Check sheet for the modelled part. Datum: model origin and axes. Units: mm. Face numbers are marked on the shaded views. Give positions to 0.01 mm unless a question says otherwise; leave off trailing zeros. Order: outer loops, then holes, each group sorted by start corner. A loop starts at its lowest first (then second) coordinate and runs counter-clockwise, first axis right, second up.
```python
from build123d import *

# Parameters (mm, degrees)
CHAMFER1_SIZE = 1
FILLET1_R     = 1


with BuildPart() as part:
    # Sketch1 → Revolve1 (revolve)
    with BuildSketch(Plane.XY, mode=Mode.PRIVATE) as revolve1_sk:
        Polygon((0, 5), (10, 5), (10, 7.5), (3, 7.5), (3, 10.5), (0, 10.5), align=None)
    revolve(revolve1_sk.sketch.rotate(Axis((0, 0, 0), (1, 0, 0)), 90), axis=Axis((0, 0, 0), (1, 0, 0)))

    # Chamfer1
    chamfer1_edges = [part.edges().sort_by_distance(p)[0] for p in [
        (0, 0, -10.5),
        (3, 0, -10.5),
        (10, 0, -7.5),
        (10, 0, -5),
        (0, 0, -5),
    ]]
    chamfer(chamfer1_edges, length=CHAMFER1_SIZE)

    # Fillet1
    fillet1_edges = [part.edges().sort_by_distance(p)[0] for p in [
        (3, 0, -7.5),
    ]]
    fillet(fillet1_edges, radius=FILLET1_R)


solid = part.part
```
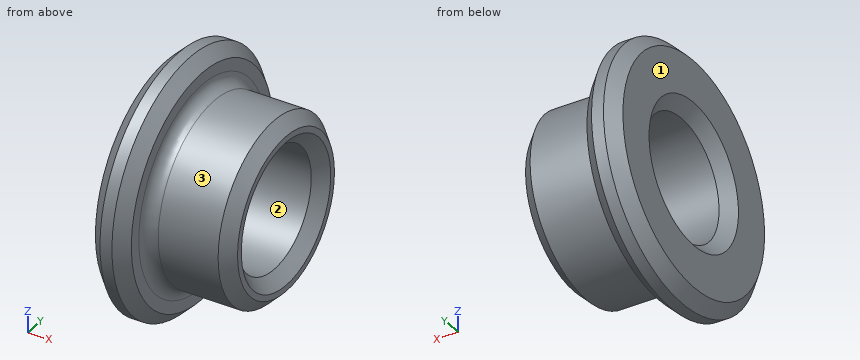
Q1. Material ranges on line 1 (Y direction, x = 1.5, z = 0); line 2 (Y direction, x = 4.5, z = 0); line 3 (X direction, y = -4.5, z = -7.25), recorded low to high.
Q2. Sectioned sample at C-C, the plane x = 2.5. Record the cut outline in (y, z), plus the area to 3 significant figures.
Q3. Sectioned sample at D-D, the plane x = 7. Record the cut outline in (y, z), plus the area to 3 significant figures.
Q4. Go/stop test with flat-tipped pins: P1, Ø6, axis at y = 0, z = 0, coming from the +X side; P2, Ø2, axis at x = 6.5, z = -2.5, coming from the +Y side; P3, Ø2, axis at x = 6.5, y = -2.5, coming from the +Z side; P4, Ø2, axis at x = 4.5, y = 1, coming from the -Z side. Record where each tip stops, or that it passes through.
Q5. Sectioned sample at A-A, the plane y = 0. Record the cut outline in (x, z), plus the area to 3 significant figures.
Q6. Draft check along Y on the marked faces 1, 2 and 3. Enter one of: pulls with the +Y half, pulls with the -Y half, needs draft (parallel to the pull), parting line crosses it, or undercut.
Filled in:
1. line 1: y = -10.5 to -5, 5 to 10.5
1. line 2: y = -7.5 to -5, 5 to 7.5
1. line 3: x = 0 to 3
2. outline: circle Ø20 at (0, 0); hole circle Ø10 at (0, 0)
2. area: 236 mm2
3. outline: circle Ø15 at (0, 0); hole circle Ø10 at (0, 0)
3. area: 98.2 mm2
4. P1: passes through
4. P2: stops at y = 7.35
4. P3: stops at z = 7.35
4. P4: stops at z = -7.58
5. outline: (0, -9.5) - (1, -10.5) - (2, -10.5) - (3, -9.5) - (3, -8.5) arc R1 cw to (4, -7.5) - (9, -7.5) - (10, -6.5) - (10, -6) - (9, -5) - (1, -5) - (0, -6) - close; (0, 6) - (1, 5) - (9, 5) - (10, 6) - (10, 6.5) - (9, 7.5) - (4, 7.5) arc R1 cw to (3, 8.5) - (3, 9.5) - (2, 10.5) - (1, 10.5) - (0, 9.5) - close
5. area: 63.4 mm2
6. face 1: needs draft
6. face 2: undercut
6. face 3: parting line crosses it
